Geometry: see drawing. Coordinates: mm, zero at the bounding-box minimum. A direction names the side the tool comes from. Round coordinates to 2 decimals unless told otherwise and drop trailing zeros. Loops run counter-clockwise (first coordinate to the right, second up) from the corner with the lowest first, then second, coordinate; pieces in that order, holes last.
(1) First-contact query: pin 1 Ø1.9 at (x, y) = (4, 41) entering from -Z; pin 2 Ø3 at (x, y) = (3, 45) entering from +Z; pin 3 Ø1.9 at (x, z) = (4.5, 32) entering from +Y. Flat tips, straight axial feed; report the tip coordinate or a pass-through.
(2) Draft query along Z for the marked faces 5, 6, 7 and 8. Return one class per face: released by +Z, released by -Z, zero draft, split by the parting line, or undercut.
(3) Cut plane D-D, the plane z = 32. Output: boundary loops of the cut face in (x, y).
(4) Line query: line 1 (Y direction, x = 2, z = 22); line 2 (Z direction, x = 1.75, y = 23.5); line 3 (Z direction, x = 2, y = 52.5). Output: solid intervals per line, ascending.
(5) Cut plane A-A, the plane z = 24. Output: boundary loops of the cut face in (x, y), and give its area (3 significant figures).
(6) Cut plane B-B, the plane x = 1.5. Output: boundary loops of the cut face in (y, z), and give its area (3 significant figures).
(7) Access query for the marked faces 1, 2, 3 and 4. Directions: +Z, -Z, +X, -X, +Y, -Y. A direction counts if a zero-diameter tool reaches every point of the face in a straight line with its end or side. Return the directions, or none.
(8) Cut plane C-C, the plane y = 43. Output: boundary loops of the cut face in (x, z).
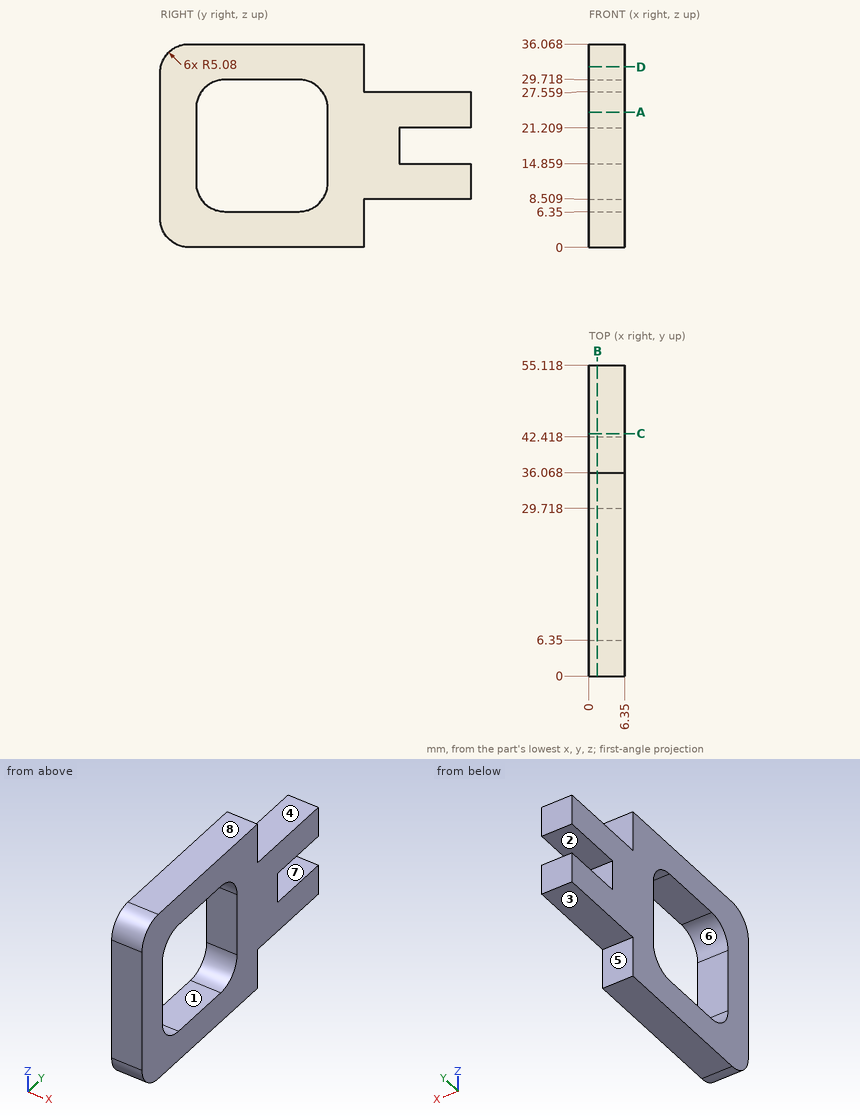
Reported:
1. pin 1: stops at z = 8.51
1. pin 2: stops at z = 27.56
1. pin 3: stops at y = 36.07
2. face 5: zero draft
2. face 6: undercut
2. face 7: undercut
2. face 8: released by +Z
3. outline: (0, 0.1) - (6.35, 0.1) - (6.35, 36.07) - (0, 36.07) - close
4. line 1: y = 0 to 6.35, 29.72 to 55.12
4. line 2: z = 0 to 6.35, 29.72 to 36.07
4. line 3: z = 8.51 to 14.86, 21.21 to 27.56
5. outline: (0, 0) - (6.35, 0) - (6.35, 6.35) - (0, 6.35) - close; (0, 29.72) - (6.35, 29.72) - (6.35, 55.12) - (0, 55.12) - close
5. area: 202 mm2
6. outline: (0, 5.08) arc R5.08 ccw to (5.08, 0) - (36.07, 0) - (36.07, 8.51) - (55.12, 8.51) - (55.12, 14.86) - (42.42, 14.86) - (42.42, 21.21) - (55.12, 21.21) - (55.12, 27.56) - (36.07, 27.56) - (36.07, 36.07) - (5.08, 36.07) arc R5.08 ccw to (0, 30.99) - close; hole (6.35, 11.43) arc R5.08 ccw to (11.43, 6.35) - (24.64, 6.35) arc R5.08 ccw to (29.72, 11.43) - (29.72, 24.64) arc R5.08 ccw to (24.64, 29.72) - (11.43, 29.72) arc R5.08 ccw to (6.35, 24.64) - close
6. area: 1,050 mm2
7. face 1: +X, -X
7. face 2: +X, -X, +Y
7. face 3: -Z, +X, -X, +Y
7. face 4: +Z, +X, -X, +Y
8. outline: (0, 8.51) - (6.35, 8.51) - (6.35, 14.86) - (0, 14.86) - close; (0, 21.21) - (6.35, 21.21) - (6.35, 27.56) - (0, 27.56) - close
